For this review, take the finished solid that the model builds, in its own axes (mm). A direction names the side the tool comes from. Coordinates: 2 decimals unless noted, no trailing zeros. Loops run counter-clockwise (first coordinate to the right, second up) from the corner with the lowest first, then second, coordinate; pieces in that order, holes last. Notation, with made-up numbers: (48, -31.75) - (67, -31.75) arc R18 cw to (67, -19.75) - close; hole circle Ø6 at (17, 36). An arc over 180 degrees is marked (long way). One line per item, written item: value. Start each with the question number.
1. Take a section at A-A, the plane z = 0. State the section outline as (x, y) points, and give its area (3 significant figures).
2. To check wall thickness, follow line 1 (X direction, y = 3.5, z = -74); line 2 (X direction, y = 4.1, z = 55); line 3 (X direction, y = 1.9, z = -15.5). State the ranges of each line that lie inside material, in increasing order. Write a range as from..to.
3. The part is to be moulded in two halves that separate along X. For faces 1 (the face through (-50.01, 2.46, -1.07)), 2 (the face through (50.01, 2.46, 1.07)), 3 (the face through (-21, 0, -1)), 4 (the face through (-67.905, 2.465, 73.133)), say which applies: released by +X, released by -X, zero draft, split by the parting line, or undercut.
4. Take a section at D-D, the plane x = -64. State the section outline as (y, z) points, and give its area (3 significant figures).
5. Insertion check: pin 1 (3 mm diameter, centred on x = 52, y = 2.5, fed in from -Z); pin 2 (6.5 mm diameter, centred on x = -64, z = 74, fed in from -Y); pin 3 (1 mm diameter, centred on y = 2.5, z = 28.5, fed in from +X); pin 4 (3 mm diameter, centred on x = -22.5, y = 2.5, fed in from +Z). Each pin has a flat end and moves straight along its axis. Give the tip position at first contact, or say it passes through.
6. Take a section at C-C, the plane x = 0. State the section outline as (y, z) points.
7. For faces 5 (the face through (61.12, 2.46, -76.78)), 6 (the face through (-0.97, 2.46, 60.01)), list the 3-axis set-ups (+Z, -Z, +X, -X, +Y, -Y) from which the entire face can be reached by the end or side of a thin tool; tool diameter is ignored.
8. Take a section at B-B, the plane y = 2.7. Count the separate pieces of the cut face and the enclosed holes in it, and give its area (3 significant figures).
```python
from build123d import *

# Parameters (mm, degrees)
SCHIZZO1_R                   = 4
ESTRUSIONE_ESTRUSIONE1_DEPTH = 5
SCHIZZO2_R                   = 1.5
TAGLIO_ESTRUSIONE1_DEPTH     = 135.629120178
SCHIZZO3_R                   = 1.5
TAGLIO_ESTRUSIONE2_DEPTH     = 135.629120178


with BuildPart() as part:
    # Schizzo1 → Estrusione-Estrusione1 (new body)
    with BuildSketch(Plane(origin=(0, 0, 0), x_dir=(1, 0, 0), z_dir=(0, 1, 0))):
        with BuildLine():
            ThreePointArc((-50, 100), (-78.284271247, 88.284271247), (-90, 60))
            ThreePointArc((-90, 60), (-50, 0), (-90, -60))
            ThreePointArc((-90, -60), (-78.284271247, -88.284271247), (-50, -100))
            ThreePointArc((-50, -100), (0, -60), (50, -100))
            ThreePointArc((50, -100), (78.284271247, -88.284271247), (90, -60))
            ThreePointArc((90, -60), (50, 0), (90, 60))
            ThreePointArc((90, 60), (78.284271247, 88.284271247), (50, 100))
            ThreePointArc((50, 100), (0, 60), (-50, 100))
        make_face()
        with Locations(Location((-64, 74, 0), (0, 0, 270))):
            Circle(SCHIZZO1_R, mode=Mode.SUBTRACT)
        with Locations(Location((-64, -74, 0), (0, 0, 270))):
            Circle(SCHIZZO1_R, mode=Mode.SUBTRACT)
        with Locations(Location((0, 0, 0), (0, 0, 270))):
            Circle(SCHIZZO1_R, mode=Mode.SUBTRACT)
        with BuildLine():
            Line((73.662823901, -78.757082536), (60.283529269, -63.891199611))
            ThreePointArc((60.283529269, -63.891199611), (54.634493757, -63.593881953), (54.337176099, -69.242917464))
            Line((54.337176099, -69.242917464), (67.716470731, -84.108800389))
            ThreePointArc((67.716470731, -84.108800389), (73.365506243, -84.406118047), (73.662823901, -78.757082536))
        make_face(mode=Mode.SUBTRACT)
        with BuildLine():
            Line((60.283529269, 63.891199611), (73.662823901, 78.757082536))
            ThreePointArc((73.662823901, 78.757082536), (73.365506243, 84.406118047), (67.716470731, 84.108800389))
            Line((67.716470731, 84.108800389), (54.337176099, 69.242917464))
            ThreePointArc((54.337176099, 69.242917464), (54.634493757, 63.593881953), (60.283529269, 63.891199611))
        make_face(mode=Mode.SUBTRACT)
    extrude(amount=ESTRUSIONE_ESTRUSIONE1_DEPTH)

    # Schizzo2 → Taglio-Estrusione1 (cut, through all)
    with BuildSketch(Plane(origin=(0, 5, 0), x_dir=(1, 0, 0), z_dir=(0, 1, 0))):
        with Locations(Location((-15.5, 15.5, 0), (0, 0, 270))):
            Circle(SCHIZZO2_R)
        with Locations(Location((15.5, 15.5, 0), (0, 0, 270))):
            Circle(SCHIZZO2_R)
        with Locations(Location((15.5, -15.5, 0), (0, 0, 270))):
            Circle(SCHIZZO2_R)
        with Locations(Location((-15.5, -15.5, 0), (0, 0, 270))):
            Circle(SCHIZZO2_R)
    extrude(amount=-TAGLIO_ESTRUSIONE1_DEPTH, mode=Mode.SUBTRACT)

    # Schizzo3 → Taglio-Estrusione2 (cut, through all)
    with BuildSketch(Plane(origin=(0, 5, 0), x_dir=(1, 0, 0), z_dir=(0, 1, 0))):
        with Locations(Location((-5, 55, 0), (0, 0, 270))):
            Circle(SCHIZZO3_R)
        with Locations(Location((5, 55, 0), (0, 0, 270))):
            Circle(SCHIZZO3_R)
        with Locations(Location((-5, -55, 0), (0, 0, 270))):
            Circle(SCHIZZO3_R)
        with Locations(Location((5, -55, 0), (0, 0, 270))):
            Circle(SCHIZZO3_R)
    extrude(amount=-TAGLIO_ESTRUSIONE2_DEPTH, mode=Mode.SUBTRACT)


solid = part.part
```
Solutions:
1. outline: (-50, 0) - (-4, 0) - (-4, 5) - (-50, 5) - close; (4, 0) - (50, 0) - (50, 5) - (4, 5) - close
1. area: 460 mm2
2. line 1: -87.47..-68, -60..-35.2, 35.2..58.62, 69.38..87.47
2. line 2: -80.36..-6.5, -3.5..3.5, 6.5..80.36
2. line 3: -51.88..-17, -14..14, 17..51.88
3. face 1: released by -X
3. face 2: released by +X
3. face 3: zero draft
3. face 4: undercut
4. outline: (0, -97.47) - (5, -97.47) - (5, -78) - (0, -78) - close; (0, -70) - (5, -70) - (5, -40.3) - (0, -40.3) - close; (0, 40.3) - (5, 40.3) - (5, 70) - (0, 70) - close; (0, 78) - (5, 78) - (5, 97.47) - (0, 97.47) - close
4. area: 492 mm2
5. pin 1: z = -100
5. pin 2: through
5. pin 3: x = 56.83
5. pin 4: z = 65.97
6. outline: (0, -60) - (5, -60) - (5, -4) - (0, -4) - close; (0, 4) - (5, 4) - (5, 60) - (0, 60) - close
7. face 5: +Y, -Y
7. face 6: +Z, +Y, -Y
8. separate pieces: 1
8. enclosed holes: 13
8. area: 21,100 mm2
